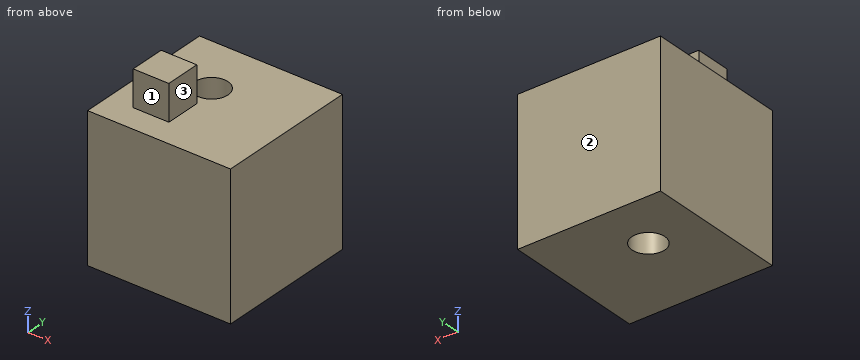
```python
from build123d import *

# Parameters (mm, degrees)
F0_W     = 101.6
F0_H     = 101.6
F1_DEPTH = 101.6
F2_R     = 11.654727
F3_DEPTH = 101.6
F4_W     = 25.4
F4_H     = 25.4
F5_DEPTH = 25.4


with BuildPart() as f1:
    # F0 (on Front) → F1 (new body)
    with BuildSketch(Plane.XZ):
        with Locations((-50.8, 50.8)):
            Rectangle(F0_W, F0_H)
    extrude(amount=F1_DEPTH)

    # F2 (on face) → F3 (cut)
    with BuildSketch(Plane.XY.offset(101.6)):
        with Locations((-61.702333, -39.977964)):
            Circle(F2_R)
    extrude(amount=-F3_DEPTH, mode=Mode.SUBTRACT)

    # F4 (on face) → F5 (join)
    with BuildSketch(Plane.XY.offset(101.6)):
        with Locations((-70.796629, -70.656015)):
            Rectangle(F4_W, F4_H)
    extrude(amount=F5_DEPTH)


solid = f1.part
```
Design review of the part built by this model. Coordinates are the model's own, in mm. Face numbers are marked on the shaded views. A direction names the side the tool comes from. Round coordinates to 2 decimals unless told otherwise and drop trailing zeros. Order: outer loops, then holes, each group sorted by start corner. A loop starts at its lowest first (then second) coordinate and runs counter-clockwise, first axis right, second up. Notation, with made-up numbers: M -14,-36 L 26,-36 A22 cw 26,1 Z; hole C 50.5,-31.5 d8. An arc over 180 degrees is marked long. Put each result on its own line as item: value.
Q1. Consider section A-A (y = -44). State the section outline as (x, z) points, and give its area (3 significant figures).
Reported:
outline: M -101.6,0 L -72.64,0 L -72.64,101.6 L -101.6,101.6 Z; M -50.76,0 L 0,0 L 0,101.6 L -50.76,101.6 Z
area: 8,100 mm²
Q2. To check wall thickness, follow line 1 (Y direction, x = -51, z = 18); line 2 (Y direction, x = -70.5, z = 120.5); line 3 (Z direction, x = -51.5, y = -97). State the ranges of each line that lie inside material, in increasing order.
Reported:
line 1: -101.6 to -44.59, -35.36 to 0
line 2: -83.36 to -57.96
line 3: 0 to 101.6
Q3. Machinability: for the marked faces 1, 2 and 3, which of the approach directions +Z, -Z, +X, -X, +Y, -Y give a long, thin tool a straight path to every point of the face, cutting with its end or side? Answer none if there is none.
Reported:
face 1: +Z, +X, -X, -Y
face 2: +Z, -Z, +X, -X, +Y
face 3: +Z, +X, +Y, -Y
Q4. Consider section D-D (z = 77.5). State the section outline as (x, y) points.
Reported:
outline: M -101.6,-101.6 L 0,-101.6 L 0,0 L -101.6,0 Z; hole C -61.7,-39.98 d23.31
Q5. Insertion check: pin 1 Ø1 at (x, y) = (-70.5, -11) entering from +Z; pin 2 Ø20.5 at (x, z) = (-75, 117) entering from +Y; pin 3 Ø21 at (x, y) = (-61.7, -39.98) entering from -Z; pin 4 Ø12.5 at (x, z) = (-74, 110.5) entering from -Y. Each pin has a flat end and moves straight along its axis. Give the tip position at first contact, or say it passes through.
Reported:
pin 1: z = 101.6
pin 2: y = -57.96
pin 3: through
pin 4: y = -83.36
Q6. Consider section B-B (y = -81). State the section outline as (x, z) points.
Reported:
outline: M -101.6,0 L 0,0 L 0,101.6 L -58.1,101.6 L -58.1,127 L -83.5,127 L -83.5,101.6 L -101.6,101.6 Z
Q7. Consider section C-C (z = 109). State the section outline as (x, y) points, and give its area (3 significant figures).
Reported:
outline: M -83.5,-83.36 L -58.1,-83.36 L -58.1,-57.96 L -83.5,-57.96 Z
area: 645 mm²
